from build123d import *

# Parameters (mm, degrees)
HOLE1_D                     = 9.525
F_1_4_20_TAPPED_HOLE1_D     = 5.1054
F_1_4_20_TAPPED_HOLE1_DEPTH = 16.51
F_1_4_20_TAPPED_HOLE1_TIP   = 1.533816902
CUT_EXTRUDE1_START          = -56.5498001
CUT_EXTRUDE1_DEPTH          = 63.8998001
CIRPATTERN1_COUNT           = 12


with BuildPart() as part:
    # Sketch1 → Revolve1 (revolve)
    with BuildSketch(Plane.XY):
        Polygon((0, 0), (0, 9.49325), (42.8498, 9.49325), (42.8498, 14.7828), (55.5498, 14.7828), (55.5498, 6.33476), (61.8998, 6.33476), (61.8998, 0), align=None)
    revolve(axis=Axis((0, 0, 0), (-1, 0, 0)))

    # Hole1 (through all)
    with Locations(Plane(origin=(10.033, 0, 9.49325), x_dir=(0, 1, 0), z_dir=(0, 0, 1))):
        with Locations((0, 0)):
            Hole(HOLE1_D / 2)

    # 1/4-20 Tapped Hole1
    with Locations(Plane(origin=(61.8998, 0, 0), x_dir=(0, 0, -1), z_dir=(1, 0, 0))):
        with Locations((0, 0)):
            Hole(F_1_4_20_TAPPED_HOLE1_D / 2, depth=F_1_4_20_TAPPED_HOLE1_DEPTH)
            with Locations((0, 0, -(F_1_4_20_TAPPED_HOLE1_DEPTH + F_1_4_20_TAPPED_HOLE1_TIP / 2))):  # 118° drill point
                Cone(0, F_1_4_20_TAPPED_HOLE1_D / 2, F_1_4_20_TAPPED_HOLE1_TIP, mode=Mode.SUBTRACT)

    # Sketch13 → Cut-Extrude1 (cut)
    with BuildSketch(Plane(origin=(55.5498, 0, 0), x_dir=(0, 0, -1), z_dir=(1, 0, 0)).offset(CUT_EXTRUDE1_START)):
        with BuildLine():
            Line((-2.852495169, 14.504980081), (-1.27, 10.157110339))
            ThreePointArc((-1.27, 10.157110339), (0, 10.2362), (1.27, 10.157110339))
            Line((1.27, 10.157110339), (2.852495169, 14.504980081))
            ThreePointArc((2.852495169, 14.504980081), (0, 14.7828), (-2.852495169, 14.504980081))
        make_face()
    cut_extrude1 = extrude(amount=CUT_EXTRUDE1_DEPTH, mode=Mode.SUBTRACT)

    # CirPattern1: Cut-Extrude1 ×12 about axis
    cirpattern1_axis = Axis((55.5498, 0, 0), (1, 0, 0))
    for i in range(1, CIRPATTERN1_COUNT):
        add(cut_extrude1.rotate(cirpattern1_axis, i * 360 / CIRPATTERN1_COUNT), mode=Mode.SUBTRACT)


solid = part.part
Geometry: final body of the model. Coordinates: model frame, mm. A direction names the side the tool comes from. Round coordinates to 2 decimals unless told otherwise and drop trailing zeros. Order: outer loops, then holes, each group sorted by start corner. A loop starts at its lowest first (then second) coordinate and runs counter-clockwise, first axis right, second up. Notation, with made-up numbers: (63.25, -28.5) - (84.25, -28.5) arc R14 ccw to (84.25, -5.5) - close; hole circle Ø1 at (-32, -14). An arc over 180 degrees is marked (long way). Write each question's results on one line, items separated by ' | '.
Item 1: Material intervals for line 1 along X through (y, z) = (0, 4); line 2 along Y through (x, z) = (44.5, -8.25); line 3 along Y through (x, z) = (58.25, 0), sorted ascending. Write a range as [from, to].
Completed:
line 1: [0, 5.27], [14.8, 61.9] | line 2: [-9.9, -6.28], [-6.06, 6.06], [6.28, 9.9] | line 3: [-6.33, -2.55], [2.55, 6.33]
Item 2: First-contact query: pin 1 Ø8 at (x, y) = (16.5, 8.5) entering from -Z; pin 2 Ø12.5 at (x, y) = (10.033, 0) entering from +Z; pin 3 Ø1 at (x, z) = (14.5, -4.5) entering from -Y. Flat tips, straight axial feed; report the tip coordinate or a pass-through.
Completed:
pin 1: z = -8.36 | pin 2: z = 9.49 | pin 3: y = -8.61
Item 3: Reachability of faces 1 (the flat face through (49.11, 2.07, -12.36)), 2 (the flat face through (49.111, 9.669, 7.975)), 3 (the cylindrical face through (21.725, 9.055, -2.852)), 4 (the cylindrical face through (49.11, -5.13, 8.86)) from +Z, -Z, +X, -X, +Y, -Y: full face, straight path, thin tool, end or side. Return the list, or none.
Completed:
face 1: -Z, +X, -X | face 2: +X, -X, +Y | face 3: -X | face 4: +X, -X
Item 4: Mould query, pull axis Z, two halves, no side actions, for faces 5 (the flat face through (49.11, -2.05, -12.3)), 6 (the conical face through (44.122, -0.17, -0.41)), 7 (the cylindrical face through (58.77, 5.85, 2.43)). Classes: pulls with the +Z half, pulls with the -Z half, needs draft (parallel to the pull), parting line crosses it, or undercut.
Completed:
face 5: pulls with the -Z half | face 6: undercut | face 7: parting line crosses it
Item 5: Section A-A, the plane z = -12. Return the cut outline in (x, y), and give its area (3 significant figures).
Completed:
outline: (42.85, -4.43) - (55.55, -4.43) - (55.55, -1.94) - (42.85, -1.94) - close; (42.85, 1.94) - (55.55, 1.94) - (55.55, 4.43) - (42.85, 4.43) - close | area: 63.3 mm^2
Item 6: Section C-C, the plane x = 42. Return the cut outline in (y, z).
Completed:
outline: circle Ø18.99 at (0, 0)
